```python
from build123d import *

# Parameters (mm, degrees)
SKETCH1_R           = 1.5875
SKETCH1_R_2         = 0.5
BOSS_EXTRUDE1_DEPTH = 5.5
SKETCH2_R           = 2
SKETCH2_R_2         = 1.5875
BOSS_EXTRUDE2_DEPTH = 0.25
SKETCH3_R           = 3
SKETCH3_R_2         = 0.5
BOSS_EXTRUDE3_DEPTH = 20
SKETCH4_R           = 1.25
CUT_EXTRUDE1_DEPTH  = 10


with BuildPart() as part:
    # Sketch1 → Boss-Extrude1 (new body)
    with BuildSketch(Plane(origin=(0, 0, 0), x_dir=(1, 0, 0), z_dir=(0, 1, 0))):
        with Locations(Location((0, 0, 0), (0, 0, 270))):
            Circle(SKETCH1_R)
        with Locations(Location((0, 0, 0), (0, 0, 270))):
            Circle(SKETCH1_R_2, mode=Mode.SUBTRACT)
    extrude(amount=BOSS_EXTRUDE1_DEPTH)

    # Sketch2 → Boss-Extrude2 (add)
    with BuildSketch(Plane(origin=(0, 5.25, 0), x_dir=(-1, 0, 0), z_dir=(0, -1, 0))):
        with Locations(Location((0, 0, 0), (0, 0, 90))):
            Circle(SKETCH2_R)
        with Locations(Location((0, 0, 0), (0, 0, 90))):
            Circle(SKETCH2_R_2, mode=Mode.SUBTRACT)
    extrude(amount=-BOSS_EXTRUDE2_DEPTH)

    # Sketch3 → Boss-Extrude3 (add)
    with BuildSketch(Plane(origin=(0, 5.5, 0), x_dir=(1, 0, 0), z_dir=(0, 1, 0))):
        with Locations(Location((0, 0, 0), (0, 0, 270))):
            Circle(SKETCH3_R)
        with Locations(Location((0, 0, 0), (0, 0, 270))):
            Circle(SKETCH3_R_2, mode=Mode.SUBTRACT)
    extrude(amount=BOSS_EXTRUDE3_DEPTH)

    # Sketch4 → Cut-Extrude1 (cut)
    with BuildSketch(Plane(origin=(0, 25.5, 0), x_dir=(1, 0, 0), z_dir=(0, 1, 0))):
        with Locations(Location((0, 0, 0), (0, 0, 270))):
            Circle(SKETCH4_R)
    extrude(amount=-CUT_EXTRUDE1_DEPTH, mode=Mode.SUBTRACT)


solid = part.part
```
Here's how the part is built. I have some questions about the finished solid (model axes, mm). A direction names the side the tool comes from. Round coordinates to 2 decimals unless told otherwise and drop trailing zeros. Order: outer loops, then holes, each group sorted by start corner. A loop starts at its lowest first (then second) coordinate and runs counter-clockwise, first axis right, second up. Notation, with made-up numbers: M 59,55.5 L 98,55.5 A21 cw 98,79.5 Z; hole C 55,-6.75 d4. An arc over 180 degrees is marked long. Use CSV: the item, a comma, the result in double quotes.
1) I need wall thicknesses on line 1 along X through (y, z) = (10, 0); line 2 along X through (y, z) = (21.5, 0); line 3 along Y through (x, z) = (-2.4, -0.8). Which ranges of each line are inside material? Lowest first, please. Write a range as [from, to].
Taken from the geometry:
line 1,"[-3, -0.5], [0.5, 3]"
line 2,"[-3, -1.25], [1.25, 3]"
line 3,"[5.5, 25.5]"
2) I'm going to push flat-ended pins straight in: P1, Ø3, axis at x = 0.5, z = 1, coming from the +Y side; P2, Ø1.5, axis at y = 11, z = 1.5, coming from the +X side. Where does each tip first touch, or does it pass through?
Taken from the geometry:
P1,"y = 25.5"
P2,"x = 2.9"
3) I want a section at C-C (y = 12.5). List the corners of the cut face in (x, z) for me, then the cut area to 3 significant figures.
Taken from the geometry:
outline,"C 0,0 d6; hole C 0,0 d1"
area,"27.5 mm^2"
4) If we mould it in two halves opening along Z, with no side actions, what happens to faces 1 (the flat face through (-1, 25.5, 1)), 2 (the cylindrical face through (-0.488, 7.642, -0.108)), 3 (the cylindrical face through (-0.966, 2.588, -1.26))? For each: pulls with the +Z half, pulls with the -Z half, needs draft (parallel to the pull), parting line crosses it, or undercut.
Taken from the geometry:
face 1,"needs draft"
face 2,"undercut"
face 3,"parting line crosses it"
5) I want a section at B-B (x = 0). List the corners of the cut face in (y, z) for me, then the cut area to 3 significant figures.
Taken from the geometry:
outline,"M 0,-1.59 L 5.25,-1.59 L 5.25,-2 L 5.5,-2 L 5.5,-3 L 25.5,-3 L 25.5,-1.25 L 15.5,-1.25 L 15.5,-0.5 L 0,-0.5 Z; M 0,0.5 L 15.5,0.5 L 15.5,1.25 L 25.5,1.25 L 25.5,3 L 5.5,3 L 5.5,2 L 5.25,2 L 5.25,1.59 L 0,1.59 Z"
area,"97.2 mm^2"
6) I want a section at D-D (z = 1). List the corners of the cut face in (x, y) for me, then the cut area to 3 significant figures.
Taken from the geometry:
outline,"M -2.83,5.5 L -1.73,5.5 L -1.73,5.25 L -1.23,5.25 L -1.23,0 L 1.23,0 L 1.23,5.25 L 1.73,5.25 L 1.73,5.5 L 2.83,5.5 L 2.83,25.5 L 0.75,25.5 L 0.75,15.5 L -0.75,15.5 L -0.75,25.5 L -2.83,25.5 Z"
area,"112 mm^2"
7) I want a section at A-A (z = 0). List the corners of the cut face in (x, y) for me.
Taken from the geometry:
outline,"M -3,5.5 L -2,5.5 L -2,5.25 L -1.59,5.25 L -1.59,0 L -0.5,0 L -0.5,15.5 L -1.25,15.5 L -1.25,25.5 L -3,25.5 Z; M 0.5,0 L 1.59,0 L 1.59,5.25 L 2,5.25 L 2,5.5 L 3,5.5 L 3,25.5 L 1.25,25.5 L 1.25,15.5 L 0.5,15.5 Z"
8) On a 3-axis mill with a long thin cutter (end or side, diameter ignored), from which of +Z, -Z, +X, -X, +Y, -Y can I reach the whole of each face in a straight line? I mean faces 4 (the flat face through (0, 0, 1)), 5 (the cylindrical face through (-1.22, 20.57, -0.27)), 6 (the flat face through (-1, 5.5, 2)). Say none if no direction works.
Taken from the geometry:
face 4,"+Z, -Z, +X, -X, -Y"
face 5,"+Y"
face 6,"-Y"
